Work out the finished part from the listing and answer in its coordinate system (mm). A direction names the side the tool comes from. Give positions to 0.01 mm unless a question says otherwise; leave off trailing zeros. Loops run counter-clockwise (first coordinate to the right, second up) from the corner with the lowest first, then second, coordinate; pieces in that order, holes last. Notation, with made-up numbers: (11, -10.5) - (41, -10.5) arc R21 ccw to (41, 2.5) - close; hole circle Ø9 at (58, 33). An arc over 180 degrees is marked (long way). One line per question, with ' | ' between items. Start each with the question number.
1. Section B-B (y = -15) is taken. Determine the outline of the cut face in (x, z), plus the area to 3 significant figures.
2. Section C-C (x = 7) is taken. Determine the outline of the cut face in (y, z) (3 decimals).
3. Section D-D (z = -1.5) is taken. Determine the outline of the cut face in (x, y) (3 decimals).
4. Each of these flat-tipped pins is pushed along its axis until it touches: pin 1 (3 mm diameter, centred on x = 18.05, y = -8.885, fed in from -Z); pin 2 (2.5 mm diameter, centred on x = 18, y = -8.5, fed in from +Z). Where does it stop, or does it pass through?
5. Which of the six approach directions +Z, -Z, +X, -X, +Y, -Y give full straight-line access (tool end or side, diameter ignored) to faces 4 (the face through (36, -9, 13)), 5 (the face through (18, -9, 0)), 6 (the face through (16.85, -8.83, 21.07))?
6. Section A-A (x = 18.05) is taken. Determine the outline of the cut face in (y, z) (3 decimals).
7. Find the intervals of material crossed by line 1 (Y direction, x = 18.05, z = 18) (3 decimals); line 2 (Z direction, x = 24, y = -12.5); line 3 (X direction, y = -8.25, z = 16.5), in increasing order.
8. For a pull along X with two mould halves and no side action, classify faces 1 (the face through (7, -9, -13.5)), 2 (the face through (18, -9, 16)), 3 (the face through (2.354, -8.681, 32.162)) as released by +X, released by -X, zero draft, split by the parting line, or undercut.
from build123d import *

# Parameters (mm, degrees)
F0_W     = 36
F0_H     = 26
F1_DEPTH = 17.77
F2_R     = 4.65
F3_DEPTH = 12.5
F2_R_2   = 1.2
F4_DEPTH = 10
F5_R     = 4.65
F6_DEPTH = 13.5


with BuildPart() as f1:
    # F0 (on Front) → F1 (new body)
    with BuildSketch(Plane.XZ):
        with Locations((18, 13)):
            Rectangle(F0_W, F0_H)
    extrude(amount=F1_DEPTH)

    # F2 (on face) → F3 (join)
    with BuildSketch(Plane.XY.offset(26)):
        with Locations((7, -8.885)):
            Circle(F2_R)
    extrude(amount=F3_DEPTH)

    # F2 (on face) → F4 (cut)
    with BuildSketch(Plane.XY.offset(26)):
        with Locations((18.05, -8.885)):
            Circle(F2_R_2)
    extrude(amount=-F4_DEPTH, mode=Mode.SUBTRACT)

    # F5 (on face) → F6 (join)
    with BuildSketch(Plane(origin=(0, 0, 0), x_dir=(1, 0, 0), z_dir=(0, 0, -1))):
        with Locations((7, 8.885)):
            Circle(F5_R)
        with Locations((29, 8.885)):
            Circle(F5_R)
    extrude(amount=F6_DEPTH)


solid = f1.part
Conclusion:
1) outline: (0, 0) - (36, 0) - (36, 26) - (0, 26) - close | area: 936 mm²
2) outline: (-17.77, 0) - (-13.535, 0) - (-13.535, -13.5) - (-4.235, -13.5) - (-4.235, 0) - (0, 0) - (0, 26) - (-4.235, 26) - (-4.235, 38.5) - (-13.535, 38.5) - (-13.535, 26) - (-17.77, 26) - close
3) outline: circle Ø9.3 at (7, -8.885); circle Ø9.3 at (29, -8.885)
4) pin 1: z = 0 | pin 2: z = 26
5) face 4: +Z, -Z, +X, +Y, -Y | face 5: -Z | face 6: +Z
6) outline: (-17.77, 0) - (0, 0) - (0, 26) - (-7.685, 26) - (-7.685, 16) - (-10.085, 16) - (-10.085, 26) - (-17.77, 26) - close
7) line 1: -17.77 to -10.085, -7.685 to 0 | line 2: 0 to 26 | line 3: 0 to 17.03, 19.07 to 36
8) face 1: zero draft | face 2: undercut | face 3: split by the parting line
